Input: part model. Units: mm. Frame: model coordinates. A direction names the side the tool comes from. Give positions to 0.01 mm unless a question says otherwise; leave off trailing zeros. Write each loop counter-clockwise with the first axis right and the second up, starting at its lowest first coordinate (ties: lowest second). Pieces come first, ordered by that corner, then holes. Notation, with made-up numbers: (77, 57) -> (133, 57) arc R23 ccw to (133, 78) -> close; hole circle Ø7 at (5.25, -15). An arc over 180 degrees is marked (long way). Return JSON: item names as keys, results as strings. Group by question number.
Item 1: Section C-C, the plane y = 17.5. Return loops of the section in (x, z).
Item 2: Set-up query: faces 1 (the face through (-7.59, -13.69, 2.46)), 2 (the face through (-1, 11, 45.6)), 3 (the face through (-8, -1, 35)). Return all of +Z, -Z, +X, -X, +Y, -Y with unobstructed straight access to the full face (end or side cutting, diameter ignored); none if empty.
Item 3: Line query: line 1 (X direction, y = -13, z = 2.5); line 2 (Y direction, x = -7.5, z = 36); line 3 (Y direction, x = 0, z = -1.8). Output: solid intervals per line, ascending. Write a range as [from, to].
Item 4: Section D-D, the plane x = -4.75. Return loops of the section in (y, z).
Item 5: Section A-A, the plane y = 10. Return loops of the section in (x, z), then the cut area to 3 significant figures.
Item 6: Pin query (flat end, axial travel): P1, Ø0.8, axis at x = -7.5, y = 17.5, coming from the +Z side; P2, Ø0.8, axis at x = 0.5, y = -17.5, coming from the -Z side; P3, Ø6, axis at x = -5, y = 10, coming from the -Z side; P4, Ø2, axis at x = -7.5, y = -1.25, coming from the +Z side. Return the tip coordinate at first contact, or that it passes through.
Item 7: Section B-B, the plane x = 0. Return loops of the section in (y, z), then the cut area to 3 significant figures.
Item 8: Mould query, pull axis X, two halves, no side actions, for faces 4 (the face through (0, 7, 43)), 5 (the face through (0, 0, 40)), 6 (the face through (-0.37, -17.86, 2.46)), 7 (the face through (8.3, -1.3, 37.5)). Classes: released by +X, released by -X, zero draft, split by the parting line, or undercut.
from build123d import *

# Parameters (mm, degrees)
SKETCH1_W           = 20.2
SKETCH1_H           = 40.2
BOSS_EXTRUDE1_DEPTH = 40
SKETCH2_R           = 0.8
CUT_EXTRUDE1_DEPTH  = 5
SKETCH3_R           = 3
SKETCH3_R_2         = 1.25
BOSS_EXTRUDE2_DEPTH = 5.6
BOSS_EXTRUDE3_START = 5.7
SKETCH4_R           = 3
SKETCH4_R_2         = 1.5
BOSS_EXTRUDE3_DEPTH = 5.7
SKETCH5_R           = 0.8
CUT_EXTRUDE2_DEPTH  = 5


with BuildPart() as part:
    # Sketch1 → Boss-Extrude1 (new body)
    with BuildSketch(Plane.XY):
        Rectangle(SKETCH1_W, SKETCH1_H)
    extrude(amount=BOSS_EXTRUDE1_DEPTH)

    # Sketch2 → Cut-Extrude1 (cut)
    with BuildSketch(Plane.XY.offset(40)):
        with Locations((-7.5, -17.5)):
            Circle(SKETCH2_R)
        with Locations(Location((-7.5, 17.5, 0), (0, 0, 180))):
            Circle(SKETCH2_R)
        with Locations(Location((7.5, -17.5, 0), (0, 0, 180))):
            Circle(SKETCH2_R)
        with Locations((7.5, 17.5)):
            Circle(SKETCH2_R)
        with Locations((-7.5, -1.25)):
            Circle(SKETCH2_R)
        with Locations(Location((7.5, -1.25, 0), (0, 0, 180))):
            Circle(SKETCH2_R)
    extrude(amount=-CUT_EXTRUDE1_DEPTH, mode=Mode.SUBTRACT)

    # Sketch3 → Boss-Extrude2 (add)
    with BuildSketch(Plane.XY.offset(40)):
        with Locations(Location((0, 10, 0), (0, 0, 180))):
            Circle(SKETCH3_R)
        with Locations((0, 10)):
            Circle(SKETCH3_R_2, mode=Mode.SUBTRACT)
    extrude(amount=BOSS_EXTRUDE2_DEPTH)

    # Sketch4 → Boss-Extrude3 (add)
    with BuildSketch(Plane(origin=(0, 0, 0), x_dir=(-1, 0, 0), z_dir=(0, 0, -1)).offset(BOSS_EXTRUDE3_START)):
        with Locations((0, 10)):
            Circle(SKETCH4_R)
        with Locations((0, 10)):
            Circle(SKETCH4_R_2, mode=Mode.SUBTRACT)
    extrude(amount=-BOSS_EXTRUDE3_DEPTH)

    # Sketch5 → Cut-Extrude2 (cut)
    with BuildSketch(Plane(origin=(0, 0, 0), x_dir=(-1, 0, 0), z_dir=(0, 0, -1))):
        with Locations((0, -17.15)):
            Circle(SKETCH5_R)
        with Locations((-7, -13.15)):
            Circle(SKETCH5_R)
        with Locations((-7, -10.15)):
            Circle(SKETCH5_R)
        with Locations(Location((7, -13.15, 0), (0, 0, 180))):
            Circle(SKETCH5_R)
        with Locations(Location((7, -10.15, 0), (0, 0, 180))):
            Circle(SKETCH5_R)
    extrude(amount=-CUT_EXTRUDE2_DEPTH, mode=Mode.SUBTRACT)


solid = part.part
Answer below:
{
 "1": {"outline": "(-10.1, 0) -> (10.1, 0) -> (10.1, 40) -> (8.3, 40) -> (8.3, 35) -> (6.7, 35) -> (6.7, 40) -> (-6.7, 40) -> (-6.7, 35) -> (-8.3, 35) -> (-8.3, 40) -> (-10.1, 40) -> close"},
 "2": {"face 1": "-Z", "face 2": "+Z, +X, -X, +Y, -Y", "face 3": "+Z"},
 "3": {"line 1": "x = [-10.1, -7.79], [-6.21, 6.21], [7.79, 10.1]", "line 2": "y = [-20.1, -18.3], [-16.7, -2.05], [-0.45, 16.7], [18.3, 20.1]", "line 3": "y = [7, 8.5], [11.5, 13]"},
 "4": {"outline": "(-20.1, 0) -> (20.1, 0) -> (20.1, 40) -> (-20.1, 40) -> close"},
 "5": {"outline": "(-10.1, 0) -> (-3, 0) -> (-3, -5.7) -> (-1.5, -5.7) -> (-1.5, 0) -> (1.5, 0) -> (1.5, -5.7) -> (3, -5.7) -> (3, 0) -> (10.1, 0) -> (10.1, 40) -> (3, 40) -> (3, 45.6) -> (1.25, 45.6) -> (1.25, 40) -> (-1.25, 40) -> (-1.25, 45.6) -> (-3, 45.6) -> (-3, 40) -> (-10.1, 40) -> close", "area": "845 mm2"},
 "6": {"P1": "stops at z = 35", "P2": "stops at z = 0", "P3": "stops at z = -5.7", "P4": "stops at z = 40"},
 "7": {"outline": "(-20.1, 0) -> (-17.95, 0) -> (-17.95, 5) -> (-16.35, 5) -> (-16.35, 0) -> (7, 0) -> (7, -5.7) -> (8.5, -5.7) -> (8.5, 0) -> (11.5, 0) -> (11.5, -5.7) -> (13, -5.7) -> (13, 0) -> (20.1, 0) -> (20.1, 40) -> (13, 40) -> (13, 45.6) -> (11.25, 45.6) -> (11.25, 40) -> (8.75, 40) -> (8.75, 45.6) -> (7, 45.6) -> (7, 40) -> (-20.1, 40) -> close", "area": "1,640 mm2"},
 "8": {"face 4": "split by the parting line", "face 5": "zero draft", "face 6": "undercut", "face 7": "undercut"}
}
